```python
from build123d import *

# Parameters (mm, degrees)
F0_W      = 50
F0_H      = 100
F0_W_2    = 42
F0_H_2    = 60
F0_H_3    = 28
F1_DEPTH  = 35
F2_W      = 50
F2_H      = 100
F3_DEPTH  = 2
F4_R      = 1.5
F5_DEPTH  = 100
F6_R      = 2.85
F7_W      = 15
F7_H      = 5
F7_H_2    = 12
F7_H_3    = 8
F7_H_4    = 23
F8_DEPTH  = 74.9
F9_W      = 42
F9_H      = 60
F9_H_2    = 28
F10_DEPTH = 0.5
F11_W     = 42
F11_H     = 2
F12_DEPTH = 34.5


with BuildPart() as f1:
    # F0 (on Top) → F1 (new body)
    with BuildSketch(Plane.XY):
        with Locations((25, 50)):
            Rectangle(F0_W, F0_H)
        with Locations((25, 34)):
            Rectangle(F0_W_2, F0_H_2, mode=Mode.SUBTRACT)
        with Locations((25, 82)):
            Rectangle(F0_W_2, F0_H_3, mode=Mode.SUBTRACT)
    extrude(amount=F1_DEPTH)

    # F2 (on face) → F3 (join)
    with BuildSketch(Plane(origin=(0, 0, 0), x_dir=(1, 0, 0), z_dir=(0, 0, -1))):
        with Locations((25, -50)):
            Rectangle(F2_W, F2_H)
    extrude(amount=F3_DEPTH)

    # F4 (on face) → F5 (join, through all)
    with BuildSketch(Plane.XZ):
        Polygon((50, 35), (50, 24.607695), (56, 35), (56, 41), (50, 41), align=None)
        with Locations((53, 38)):
            Circle(F4_R, mode=Mode.SUBTRACT)
    extrude(amount=-F5_DEPTH)

    # F6
    f6_edges = [f1.edges().sort_by_distance(p)[0] for p in [
        (56, 50, 41),
        (50, 50, 41),
    ]]
    fillet(f6_edges, radius=F6_R)

    # F7 (on face) → F8 (cut)
    with BuildSketch(Plane(origin=(0, 0, -2), x_dir=(1, 0, 0), z_dir=(0, 0, -1))):
        with Locations((57.5, -2.5)):
            Rectangle(F7_W, F7_H)
        with Locations((57.5, -66)):
            Rectangle(F7_W, F7_H_2)
        with Locations((57.5, -96)):
            Rectangle(F7_W, F7_H_3)
        with Locations((57.5, -82)):
            Rectangle(F7_W, F7_H_2)
        with Locations((57.5, -52)):
            Rectangle(F7_W, F7_H_3)
        with Locations((57.5, -13)):
            Rectangle(F7_W, F7_H_3)
        with Locations((57.5, -32.5)):
            Rectangle(F7_W, F7_H_4)
    extrude(amount=-F8_DEPTH, mode=Mode.SUBTRACT)

    # F9 (on face) → F10 (cut)
    with BuildSketch(Plane.XY.offset(35)):
        Polygon((0, 100), (0, 0), (50, 0), (50, 5), (50, 9), (50, 17), (50, 21), (50, 44), (50, 48), (50, 56), (50, 60), (50, 72), (50, 76), (50, 88), (50, 92), (50, 100), align=None)
        with Locations((25, 34)):
            Rectangle(F9_W, F9_H, mode=Mode.SUBTRACT)
        with Locations((25, 82)):
            Rectangle(F9_W, F9_H_2, mode=Mode.SUBTRACT)
    extrude(amount=-F10_DEPTH, mode=Mode.SUBTRACT)

    # F11 (on face) → F12 (join, through all)
    with BuildSketch(Plane.XY.offset(34.5)):
        with Locations((25, 33)):
            Rectangle(F11_W, F11_H)
    extrude(amount=-F12_DEPTH)


solid = f1.part
```
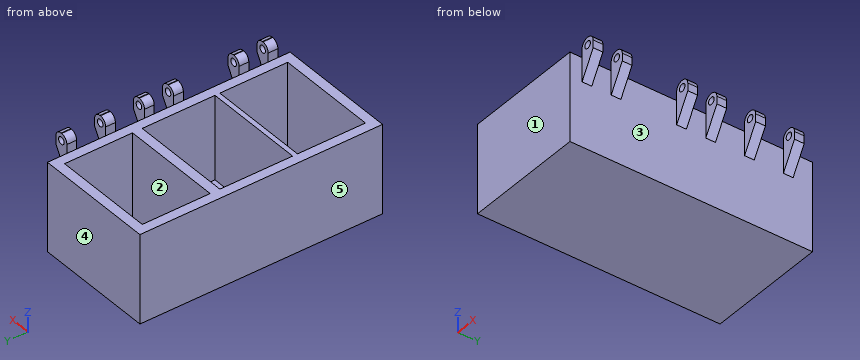
Input: part model. Units: mm. Frame: model coordinates. Face numbers are marked on the shaded views. A direction names the side the tool comes from. Give positions to 0.01 mm unless a question says otherwise; leave off trailing zeros. Loops run counter-clockwise (first coordinate to the right, second up) from the corner with the lowest first, then second, coordinate; pieces in that order, holes last. Notation, with made-up numbers: M 58.25,15.5 L 77.25,15.5 A29 ccw 77.25,45.5 Z; hole C -11,-11.5 d9. An arc over 180 degrees is marked long. Answer as CSV lines item,"result". Start each with the question number.
1. Line query: L1, parallel to Y at x = 33, z = 17; L2, parallel to Y at x = 51, z = 38; L3, parallel to X at y = 51, z = 32. Output: solid intervals per line, ascending.
2. Reachability of the marked faces 1 and 2 from +Z, -Z, +X, -X, +Y, -Y: full face, straight path, thin tool, end or side. Return the list, or none.
3. Section B-B on y = 39.5. Return loops of the section in (x, z), plus the area to 3 significant figures.
4. Section A-A on z = 8. Return loops of the section in (x, y).
5. Pull-direction query (Y, two-part tool) for the marked faces 3, 4 and 5; classes: released by +Y, released by -Y, zero draft, split by the parting line, or undercut.
6. Section C-C on x = 5.5. Return loops of the section in (y, z), plus the area to 3 significant figures.
7. Pin query (flat end, axial travel): P1, Ø2, axis at x = 12.5, y = 25, coming from the +Z side; P2, Ø1.8, axis at x = 53, z = 38, coming from the +Y side; P3, Ø8.5, axis at y = 11.5, z = 16.5, coming from the +X side; P4, Ø3, axis at y = 91, z = 36.5, coming from the -X side. Return the tip coordinate at first contact, or that it passes through.
Computed values:
1,L1,"y = 0 to 4, 32 to 34, 64 to 68, 96 to 100"
1,L2,"y = 5 to 9, 17 to 21, 44 to 48, 56 to 60, 72 to 76, 88 to 92"
1,L3,"x = 0 to 4, 46 to 50"
2,face 1,"+Z, -Z, +X, -X, -Y"
2,face 2,"+Z"
3,outline,"M 0,-2 L 50,-2 L 50,34.5 L 46,34.5 L 46,0 L 4,0 L 4,34.5 L 0,34.5 Z"
3,area,"376 mm²"
4,outline,"M 0,0 L 50,0 L 50,100 L 0,100 Z; hole M 4,4 L 46,4 L 46,32 L 4,32 Z; hole M 4,34 L 46,34 L 46,64 L 4,64 Z; hole M 4,68 L 46,68 L 46,96 L 4,96 Z"
5,face 3,"undercut"
5,face 4,"released by +Y"
5,face 5,"zero draft"
6,outline,"M 0,-2 L 100,-2 L 100,34.5 L 96,34.5 L 96,0 L 68,0 L 68,34.5 L 64,34.5 L 64,0 L 34,0 L 34,34.5 L 32,34.5 L 32,0 L 4,0 L 4,34.5 L 0,34.5 Z"
6,area,"683 mm²"
7,P1,"stops at z = 0"
7,P2,"passes through"
7,P3,"stops at x = 50"
7,P4,"stops at x = 50"
